```python
from build123d import *

# Parameters (mm, degrees)
SKETCH_1_W           = 44
SKETCH_1_H           = 25
SKETCH_1_W_2         = 40.6
SKETCH_1_H_2         = 21.6
EXTRUDE_1_DEPTH      = 44.2
SKETCH_2_W           = 5.55
SKETCH_2_H           = 25
EXTRUDE_2_DEPTH      = 10
SKETCH_3_W           = 44
SKETCH_3_H           = 21.6
CUT_EXTRUDE_1_DEPTH  = 13.2
SKETCH_4_R           = 2
CUT_EXTRUDE_2_DEPTH  = 10
FILLET_1_R           = 2
SKETCH_5_W           = 44
SKETCH_5_H           = 44.2
EXTRUDE_3_DEPTH      = 6
SKETCH_9_R           = 1
EXTRUDE_4_DEPTH      = 2
EXTRUDE_5_DEPTH      = 1.5
SKETCH_12_R          = 35.05
SKETCH_12_R_2        = 32.9
CUT_EXTRUDE_6_DEPTH  = 1
SKETCH_13_R          = 1.5
CUT_EXTRUDE_7_DEPTH  = 30
SKETCH_14_W          = 2
SKETCH_14_H          = 12
CUT_EXTRUDE_8_DEPTH  = 25
FILLET_2_R           = 8
SKETCH_16_R          = 7.216878365
CUT_EXTRUDE_10_DEPTH = 10
FILLET_3_R           = 4
CUT_EXTRUDE_11_REACH = 107.631
SKETCH_17_W          = 44
SKETCH_17_H          = 2
SKETCH_21_W          = 227.693891034
SKETCH_21_H          = 191.913422443
CUT_EXTRUDE_15_DEPTH = 16
CUT_EXTRUDE_17_DEPTH = 10
SKETCH_31_W          = 40
SKETCH_31_H          = 38.2
EXTRUDE_10_DEPTH     = 3
CUT_EXTRUDE_18_DEPTH = 2


with BuildPart() as part:
    # 草图1 → 凸台-拉伸1 (new body)
    with BuildSketch(Plane.XY):
        Rectangle(SKETCH_1_W, SKETCH_1_H)
        Rectangle(SKETCH_1_W_2, SKETCH_1_H_2, mode=Mode.SUBTRACT)
    extrude(amount=-EXTRUDE_1_DEPTH)

    # 草图2 → 凸台-拉伸2 (add)
    with BuildSketch(Plane(origin=(0, 0, -13.2), x_dir=(-1, 0, 0), z_dir=(0, 0, -1))):
        with Locations((-24.775, 0)):
            Rectangle(SKETCH_2_W, SKETCH_2_H)
        with Locations((24.775, 0)):
            Rectangle(SKETCH_2_W, SKETCH_2_H)
    extrude(amount=EXTRUDE_2_DEPTH)

    # 草图3 → 切除-拉伸1 (cut)
    with BuildSketch(Plane.XY):
        Rectangle(SKETCH_3_W, SKETCH_3_H)
    extrude(amount=-CUT_EXTRUDE_1_DEPTH, mode=Mode.SUBTRACT)

    # 草图4 → 切除-拉伸2 (cut)
    with BuildSketch(Plane.XY.offset(-13.2)):
        with Locations((24, 5)):
            Circle(SKETCH_4_R)
        with Locations((24, -5)):
            Circle(SKETCH_4_R)
        with Locations((-24, 5)):
            Circle(SKETCH_4_R)
        with Locations((-24, -5)):
            Circle(SKETCH_4_R)
    extrude(amount=-CUT_EXTRUDE_2_DEPTH, mode=Mode.SUBTRACT)

    # 圆角1
    fillet_1_edges = [part.edges().sort_by_distance(p)[0] for p in [
        (27.55, 12.5, -18.2),
        (27.55, -12.5, -18.2),
    ]]
    fillet(fillet_1_edges, radius=FILLET_1_R)

    # 草图5 → 凸台-拉伸3 (add)
    with BuildSketch(Plane.XZ.offset(12.5)):
        with Locations((0, -22.1)):
            Rectangle(SKETCH_5_W, SKETCH_5_H)
    extrude(amount=EXTRUDE_3_DEPTH)

    # 草图9 → 凸台-拉伸4 (add)
    with BuildSketch(Plane.XZ.offset(18.5)):
        Polygon((-46.27864045, -52.2), (33.72135955, -52.2), (58.4427191, 23.884521304), (-6.27864045, 70.907341487), (-71, 23.884521304), align=None)
        with Locations(Location((-6.27864045, 2.855276819, 0), (0, 0, 270))):
            Circle(SKETCH_9_R, mode=Mode.SUBTRACT)
    extrude(amount=EXTRUDE_4_DEPTH)

    # 草图10 → 凸台-拉伸5 (add)
    with BuildSketch(Plane(origin=(0, -18.5, 0), x_dir=(1, 0, 0), z_dir=(0, 1, 0))):
        Polygon((-64.534362225, -21.783708242), (-6.27864045, -64.108967611), (51.977081325, -21.783708242), (29.725375646, 46.7), (-42.282656546, 46.7), align=None)
        Polygon((-62.183221216, -21.019776219), (-6.27864045, -61.636831656), (49.625940316, -21.019776219), (28.27229059, 44.7), (-40.82957149, 44.7), align=None, mode=Mode.SUBTRACT)
    extrude(amount=EXTRUDE_5_DEPTH)

    # 草图12 → 切除-拉伸6 (cut)
    with BuildSketch(Plane.XZ.offset(20.5)):
        with Locations(Location((-6.27864045, 2.855276819, 0), (0, 0, 270))):
            Circle(SKETCH_12_R)
        with Locations(Location((-6.27864045, 2.855276819, 0), (0, 0, 270))):
            Circle(SKETCH_12_R_2, mode=Mode.SUBTRACT)
    extrude(amount=-CUT_EXTRUDE_6_DEPTH, mode=Mode.SUBTRACT)

    # 草图13 → 切除-拉伸7 (cut)
    with BuildSketch(Plane.XZ.offset(20.5)):
        with Locations(Location((-6.27864045, 65.855276819, 0), (0, 0, 270))):
            Circle(SKETCH_13_R)
        with Locations(Location((53.637920077, 22.323347464, 0), (0, 0, 270))):
            Circle(SKETCH_13_R)
        with Locations(Location((30.751830444, -48.112793827, 0), (0, 0, 270))):
            Circle(SKETCH_13_R)
        with Locations(Location((-43.309111344, -48.112793827, 0), (0, 0, 270))):
            Circle(SKETCH_13_R)
        with Locations(Location((-66.195200977, 22.323347464, 0), (0, 0, 270))):
            Circle(SKETCH_13_R)
    extrude(amount=-CUT_EXTRUDE_7_DEPTH, mode=Mode.SUBTRACT)

    # 草图14 → 切除-拉伸8 (cut)
    with BuildSketch(Plane.XY.offset(-13.2)):
        with Locations((21.3, 0)):
            Rectangle(SKETCH_14_W, SKETCH_14_H)
    extrude(amount=-CUT_EXTRUDE_8_DEPTH, mode=Mode.SUBTRACT)

    # 圆角2
    fillet_2_edges = [part.edges().sort_by_distance(p)[0] for p in [
        (-22, 11.65, 0),
        (22, 11.65, 0),
    ]]
    fillet(fillet_2_edges, radius=FILLET_2_R)

    # 草图16 → 切除-拉伸10 (cut)
    with BuildSketch(Plane(origin=(0, -18.5, 0), x_dir=(1, 0, 0), z_dir=(0, 1, 0))):
        with Locations(Location((-14.634879376, -12.813854579, 0), (0, 0, 270))):
            Circle(SKETCH_16_R)
    extrude(amount=-CUT_EXTRUDE_10_DEPTH, mode=Mode.SUBTRACT)

    # 圆角3
    fillet_3_edges = [part.edges().sort_by_distance(p)[0] for p in [
        (-22, -14.65, 0),
        (22, -14.65, 0),
    ]]
    fillet(fillet_3_edges, radius=FILLET_3_R)

    # 切除-拉伸11: up to this face of the body (flat: up to its plane)
    cut_extrude_11_end = Plane(part.part.faces().sort_by_distance((23.543010381, -18.5, -24.1))[0])
    # 草图17 → 切除-拉伸11 (cut, up to the picked face)
    with BuildSketch(Plane(origin=(0, 12.5, 0), x_dir=(1, 0, 0), z_dir=(0, 1, 0)), mode=Mode.PRIVATE) as cut_extrude_11_sk1:
        with Locations((0, 43.2)):
            Rectangle(SKETCH_17_W, SKETCH_17_H)
    cut_extrude_11_tool1 = split(extrude(cut_extrude_11_sk1.sketch, amount=-CUT_EXTRUDE_11_REACH, mode=Mode.PRIVATE), bisect_by=cut_extrude_11_end, keep=Keep.BOTH, mode=Mode.PRIVATE)
    add(cut_extrude_11_tool1.solids().sort_by(Axis((0, 12.5, -43.2), (0, -1, 0)))[0], mode=Mode.SUBTRACT)

    # 草图21 → 切除-拉伸15 (cut)
    with BuildSketch(Plane(origin=(0, -15.5, 0), x_dir=(1, 0, 0), z_dir=(0, 1, 0))):
        with Locations((-2.520580865, -1.129519683)):
            Rectangle(SKETCH_21_W, SKETCH_21_H)
    extrude(amount=-CUT_EXTRUDE_15_DEPTH, mode=Mode.SUBTRACT)

    # 草图25 → 切除-拉伸17 (cut)
    with BuildSketch(Plane(origin=(0, -10.8, 0), x_dir=(1, 0, 0), z_dir=(0, 1, 0))):
        with BuildLine():
            Line((-22, 5), (-22, 0))
            Line((-22, 0), (-17, 0))
            ThreePointArc((-17, 0), (-20.535533906, 1.464466094), (-22, 5))
        make_face()
    extrude(amount=-CUT_EXTRUDE_17_DEPTH, mode=Mode.SUBTRACT)

    # 草图31 → 凸台-拉伸10 (add)
    with BuildSketch(Plane.XZ.offset(15.5)):
        with Locations((0, -21.1)):
            Rectangle(SKETCH_31_W, SKETCH_31_H)
    extrude(amount=EXTRUDE_10_DEPTH)

    # 草图32 → 切除-拉伸18 (cut)
    with BuildSketch(Plane(origin=(0, 12.5, 0), x_dir=(1, 0, 0), z_dir=(0, 1, 0))):
        Polygon((-10.5, 37.2), (-15, 32.7), (-15, 28.2), (-6, 37.2), align=None)
        Polygon((-1.5, 37.2), (-15, 23.7), (-15, 19.2), (3, 37.2), align=None)
        Polygon((7.5, 37.2), (-15, 14.7), (-15, 10.2), (12, 37.2), align=None)
        Polygon((-7.5, 7.2), (-12, 7.2), (15, 34.2), (15, 29.7), align=None)
        Polygon((1.5, 7.2), (-3, 7.2), (15, 25.2), (15, 20.7), align=None)
        Polygon((15, 16.2), (15, 11.7), (10.5, 7.2), (6, 7.2), align=None)
    extrude(amount=-CUT_EXTRUDE_18_DEPTH, mode=Mode.SUBTRACT)


solid = part.part
```
Design review of the part built by this model. Coordinates are the model's own, in mm. A direction names the side the tool comes from. Coordinates: 2 decimals unless noted, no trailing zeros. Order: outer loops, then holes, each group sorted by start corner. A loop starts at its lowest first (then second) coordinate and runs counter-clockwise, first axis right, second up. Notation, with made-up numbers: M -29,7.5 L 13,7.5 A32 cw 13,37.5 Z; hole C -8.75,2 d1. An arc over 180 degrees is marked long. Answer as a JSON object with one key per item and string values. Group by question number.
1) Mouldability with a two-part tool opening along Z and no side actions: class faces 1 (the flat face through (22.3, 0, -18)), 2 (the flat face through (5.9, 11.7, -16.1)), 3 (the cylindrical face through (20.859, -13.117, -1.203)) as pulls with the +Z half, pulls with the -Z half, needs draft (parallel to the pull), parting line crosses it, or undercut.
2) Add section A-A, the plane z = -26. Write out the cut boundary in (x, y), then the cut area to 3 significant figures.
3) Add section C-C, the plane y = 8.5. Write out the cut boundary in (x, z).
4) Add section B-B, the plane x = 4. Write out the cut boundary in (y, z), then the cut area to 3 significant figures.
5) Tool access review of faces 4 (the flat face through (3.9, 11.7, -18.6)), 5 (the cylindrical face through (-19.719, 11.662, -2.406)), 6 (the cylindrical face through (19.594, 11.662, -2.281)), 7 (the flat face through (27.55, 0, -18)), 8 (the flat face through (24, -12.5, -18)): name each direction out of +Z, -Z, +X, -X, +Y, -Y from which nothing blocks a thin tool from reaching the whole face with its end or side.
6) Add section D-D, the plane x = -24. Write out the cut boundary in (y, z), then the cut area to 3 significant figures.
7) Wall thickness on L1, parallel to Y at x = -24, z = -15.25; L2, parallel to Y at x = 8.5, z = -39.5; L3, parallel to X at y = 6.5, z = -28: over which ranges is each line inside the solid? List them lowest first.
8) For pin 1 (4.5 mm diameter, centred on x = -24.5, z = -18, fed in from -Y); pin 2 (1.4 mm diameter, centred on y = 11.5, z = -30.5, fed in from +X); pin 3 (1.9 mm diameter, centred on x = 21.5, y = -2.5, fed in from +Z), all flat-tipped, find the tip position at first contact; note any pin that passes through.
Computed values:
{
 "1": {"face 1": "needs draft", "face 2": "undercut", "face 3": "pulls with the +Z half"},
 "2": {"outline": "M -22,-15.5 L -20,-15.5 L -20,-18.5 L 20,-18.5 L 20,-15.5 L 22,-15.5 L 22,-6 L 20.3,-6 L 20.3,-10.8 L -20.3,-10.8 L -20.3,10.8 L -12.7,10.8 L -12.7,12.5 L -22,12.5 Z; M -8.2,10.8 L -3.7,10.8 L -3.7,12.5 L -8.2,12.5 Z; M 0.8,10.8 L 6.8,10.8 L 6.8,12.5 L 0.8,12.5 Z; M 11.3,10.8 L 20.3,10.8 L 20.3,6 L 22,6 L 22,12.5 L 11.3,12.5 Z", "area": "432 mm^2"},
 "3": {"outline": "M -27.55,-23.2 L -22,-23.2 L -22,-42.2 L -20.3,-42.2 L -20.3,-13.2 L -27.55,-13.2 Z; M 20.3,-42.2 L 22,-42.2 L 22,-23.2 L 27.55,-23.2 L 27.55,-13.2 L 20.3,-13.2 Z"},
 "4": {"outline": "M -18.5,-40.2 L -15.5,-40.2 L -15.5,-42.2 L -10.8,-42.2 L -10.8,0 L -15.5,0 L -15.5,-2 L -18.5,-2 Z; M 10.8,-42.2 L 12.5,-42.2 L 12.5,-33.7 L 10.8,-33.7 Z; M 10.8,-29.2 L 12.5,-29.2 L 12.5,-23.2 L 10.8,-23.2 Z; M 10.8,-18.7 L 12.5,-18.7 L 12.5,-14.2 L 10.8,-14.2 Z; M 10.8,-9.7 L 12.5,-9.7 L 12.5,0 L 10.8,0 Z", "area": "362 mm^2"},
 "5": {"face 4": "+Y", "face 5": "+Z, -X, +Y", "face 6": "+Z, +X, +Y", "face 7": "+Z, -Z, +X, +Y, -Y", "face 8": "+Z, -Z, +X, -Y"},
 "6": {"outline": "M -12.5,-23.2 L -7,-23.2 L -7,-13.2 L -12.5,-13.2 Z; M -3,-23.2 L 3,-23.2 L 3,-13.2 L -3,-13.2 Z; M 7,-23.2 L 12.5,-23.2 L 12.5,-13.2 L 7,-13.2 Z", "area": "170 mm^2"},
 "7": {"L1": "y = -12.5 to -7, -3 to 3, 7 to 12.5", "L2": "y = -18.5 to -10.8, 10.8 to 12.5", "L3": "x = -22 to -20.3, 20.3 to 22"},
 "8": {"pin 1": "stops at y = -12.5", "pin 2": "stops at x = 22", "pin 3": "stops at z = -13.2"}
}
